Could you check a few things on this model? Use its own coordinates, in mm. A direction names the side the tool comes from. Give positions to 0.01 mm unless a question says otherwise; leave off trailing zeros. Order: outer loops, then holes, each group sorted by start corner. A loop starts at its lowest first (then second) coordinate and runs counter-clockwise, first axis right, second up.
from build123d import *

# Parameters (mm, degrees)
F0_W      = 120
F0_H      = 64
F1_DEPTH  = 25
F3_DEPTH  = 64.001
F5_DEPTH  = 64.001
F7_DEPTH  = 120.001
F8_T      = -2
F9_R      = 3.259803
F10_DEPTH = 25
F12_DEPTH = 3.5
F13_SIZE  = 2
F14_R     = 6


with BuildPart() as f1:
    # F0 (on Top) → F1 (new body)
    with BuildSketch(Plane.XY):
        Rectangle(F0_W, F0_H)
    extrude(amount=F1_DEPTH)

    # F2 (on face) → F3 (cut, through all)
    with BuildSketch(Plane.XZ.offset(32)):
        Polygon((60, 25), (-60, 25), (60, 15), align=None)
    extrude(amount=-F3_DEPTH, mode=Mode.SUBTRACT)

    # F4 (on face) → F5 (cut, through all)
    with BuildSketch(Plane.XZ.offset(32)):
        Polygon((50.034542, 15.830455), (60, 0), (60, 15), align=None)
    extrude(amount=-F5_DEPTH, mode=Mode.SUBTRACT)

    # F6 (on face) → F7 (cut, through all)
    with BuildSketch(Plane(origin=(-60, 0, 0), x_dir=(0, -1, 0), z_dir=(-1, 0, 0))):
        Polygon((-27, 25), (-32, 25), (-32, 0), align=None)
        Polygon((32, 25), (27, 25), (32, 0), align=None)
    extrude(amount=-F7_DEPTH, mode=Mode.SUBTRACT)

    # F8
    f8_openings = [f1.faces().sort_by_distance(p)[0] for p in [
        (0, 0, 0),
    ]]
    offset(amount=F8_T, openings=f8_openings)

    # F9 (on face) → F10 (cut)
    with BuildSketch(Plane(origin=(-60, 0, 0), x_dir=(0, -1, 0), z_dir=(-1, 0, 0))):
        Circle(F9_R)
    extrude(amount=-F10_DEPTH, mode=Mode.SUBTRACT)

    # F11 (on face) → F12 (join)
    with BuildSketch(Plane(origin=(0, 0, 0), x_dir=(1, 0, 0), z_dir=(0, 0, -1))):
        Polygon((-51, 29.960392), (-58, 29.960392), (-58, 22.960392), align=None)
        Polygon((57.63671, 22.587352), (57.63671, 29.960392), (50.568968, 29.960392), align=None)
        Polygon((57.63671, -22.587352), (50.568968, -29.960392), (57.63671, -29.960392), align=None)
        Polygon((-58, -22.960392), (-58, -29.960392), (-51, -29.960392), align=None)
    extrude(amount=-F12_DEPTH)

    # F13
    f13_edges = [f1.edges().sort_by_distance(p)[0] for p in [
        (-54.85, 26.110392, 3.5),
        (53.336701, -27.073104, 3.5),
        (-54.85, -26.110392, 3.5),
        (53.336701, 27.073104, 3.5),
    ]]
    chamfer(f13_edges, length=F13_SIZE)

    # F14
    f14_edges = [f1.edges().sort_by_distance(p)[0] for p in [
        (55.017271, -30.416955, 7.915227),
        (55.017271, 30.416955, 7.915227),
        (-60, -29.5, 12.5),
        (-60, 29.5, 12.5),
    ]]
    fillet(f14_edges, radius=F14_R)


solid = f1.part
Item 1: Imagine slicing it at A-A on y = 0. List the corners of the cut face in (x, z) for me.
Findings:
outline: (-60, 3.26) - (-58, 3.26) - (-58, 22.83) - (48.87, 13.92) - (57.64, 0) - (60, 0) - (50.03, 15.83) - (-60, 25) - close
Item 2: Imagine slicing it at B-B on x = 1.5. List the corners of the cut face in (y, z) for me (3 decimals).
Findings:
outline: (-32, 0) - (-29.96, 0) - (-26.387, 17.868) - (26.387, 17.868) - (29.96, 0) - (32, 0) - (28.025, 19.875) - (-28.025, 19.875) - close
Item 3: We'd pull the mould along X, two halves only. Please class faces 1 (the flat face through (-57, -28, 3.5)), 2 (the cylindrical face through (-59.01, -0.07, 3.26)), 3 (the cylindrical face through (52.744, -28.644, 8.711)): +X half, -X half, draft (parallel to the pull), parting line (faces both ways), or undercut.
Findings:
face 1: undercut
face 2: draft
face 3: +X half
Item 4: Please list where these lines run through material, in increasing order: line 1 along X through (y, z) = (-20, 6.75); line 2 along Y through (x, z) = (-23.5, 17); line 3 along X through (y, z) = (-1, 9.5).
Findings:
line 1: x = -60 to -58, 53.39 to 55.75
line 2: y = -28.6 to -26.56, 26.56 to 28.6
line 3: x = -60 to -58, 51.66 to 54.02
Item 5: For pin 1 (1 mm diameter, centred on x = 2, y = 21, fed in from +Z) (3 decimals); pin 2 (0.7 mm diameter, centred on x = 54.5, y = 28.5, fed in from +Z); pin 3 (1.5 mm diameter, centred on x = -19.5, y = -24, fed in from +Z), each with a flat end and sliding along its axis, tell me the tip position at first contact or that it passes through.
Findings:
pin 1: stops at z = 19.875
pin 2: stops at z = 7.33
pin 3: stops at z = 21.69
Item 6: For faces 4 (the flat face through (-57, 28, 3.5)), 5 (the cylindrical face through (-58.289, 27.576, 12.918)), 6 (the flat face through (-54.55, -26.41, 0.74)), which set-ups out of +Z, -Z, +X, -X, +Y, -Y let a thin tool reach every point of the face, with its end or its side?
Findings:
face 4: none
face 5: +Z, -X, +Y
face 6: -Z
